```python
from build123d import *

# Parameters (mm, degrees)
SKETCH_1_R               = 28.5
SKETCH_1_R_2             = 21.75
EXTRUDE_1_DEPTH          = 8
CHAMFER_1_SIZE           = 1
CHAMFER_2_SIZE           = 0.5
CUT_EXTRUDE_START        = -8
CUT_EXTRUDE_1_DEPTH      = 8
PATTERN_CIRCULAR_1_COUNT = 4


with BuildPart() as part:
    # 草图1 → 凸台-拉伸1 (new body)
    with BuildSketch(Plane(origin=(0, 0, 0), x_dir=(0, 0, -1), z_dir=(1, 0, 0))):
        Circle(SKETCH_1_R)
        Circle(SKETCH_1_R_2, mode=Mode.SUBTRACT)
    extrude(amount=EXTRUDE_1_DEPTH)

    # 倒角1
    chamfer_1_edges = [part.edges().sort_by_distance(p)[0] for p in [
        (0, 0, 21.75),
        (8, 0, 21.75),
    ]]
    chamfer(chamfer_1_edges, length=CHAMFER_1_SIZE)

    # 倒角2
    chamfer_2_edges = [part.edges().sort_by_distance(p)[0] for p in [
        (0, 0, 28.5),
    ]]
    chamfer(chamfer_2_edges, length=CHAMFER_2_SIZE)

    # 草图2 → 切除-拉伸1 (cut)
    with BuildSketch(Plane(origin=(8, 0, 0), x_dir=(0, 0, -1), z_dir=(1, 0, 0)).offset(CUT_EXTRUDE_START)):
        with BuildLine():
            Line((-3, 28.341665442), (-3, 26.5))
            Line((-3, 26.5), (3, 26.5))
            Line((3, 26.5), (3, 28.341665442))
            ThreePointArc((3, 28.341665442), (0, 28.5), (-3, 28.341665442))
        make_face()
    cut_extrude_1 = extrude(amount=CUT_EXTRUDE_1_DEPTH, mode=Mode.SUBTRACT)

    # 阵列(圆周)1: 切除-拉伸1 ×4 about axis
    pattern_circular_1_axis = Axis((0, 0, 0), (1, 0, 0))
    for i in range(1, PATTERN_CIRCULAR_1_COUNT):
        add(cut_extrude_1.rotate(pattern_circular_1_axis, i * 360 / PATTERN_CIRCULAR_1_COUNT), mode=Mode.SUBTRACT)

    # 草图3 → 切除-旋转1 (revolve, cut)
    with BuildSketch(Plane.XY, mode=Mode.PRIVATE) as cut_revolve_1_sk:
        Polygon((3.295131606, 35.18962283), (8, 25.1), (8, 35.18962283), align=None)
    revolve(cut_revolve_1_sk.sketch.rotate(Axis((8, 0, 0), (-1, 0, 0)), 276.042328419), axis=Axis((8, 0, 0), (-1, 0, 0)), mode=Mode.SUBTRACT)


solid = part.part
```
For this review, take the finished solid that the model builds, in its own axes (mm). A direction names the side the tool comes from. Give positions to 0.01 mm unless a question says otherwise; leave off trailing zeros. Order: outer loops, then holes, each group sorted by start corner. A loop starts at its lowest first (then second) coordinate and runs counter-clockwise, first axis right, second up.
1) Take a section at A-A (z = 0). Give the boundary of the cut face in (x, y).
2) Take a section at C-C (x = 3). Give the boundary of the cut face in (y, z), then the cut area to 3 significant figures.
3) The part is to be moulded in two halves that separate along Z. For faces 5 (the face through (4, 3, -27)), 6 (the face through (4, -26.5, 0)), 7 (the face through (3.416, 19.96, -20.343)), say which applies: released by +Z, released by -Z, zero draft, split by the parting line, or undercut.
4) Wall thickness on line 1 (Y direction, x = 5.4, z = 0); line 2 (Z direction, x = 6, y = 20); line 3 (Z direction, x = 2.5, y = 3.5): over which ranges is each line inside the solid? List them lowest first.
5) For faces 1 (the face through (4, -3, 27)), 2 (the face through (4, -3, -27)), 3 (the face through (4, -27, 3)), 4 (the face through (4, 26.5, 0)), list the 3-axis set-ups (+Z, -Z, +X, -X, +Y, -Y) from which the entire face can be reached by the end or side of a thin tool; tool diameter is ignored.
6) Insertion check: pin 1 (3 mm diameter, centred on x = 3, z = 0.5, fed in from -Y); pin 2 (1.8 mm diameter, centred on x = 2, y = 1.5, fed in from +Z); pin 3 (2 mm diameter, centred on x = 2, y = 27, fed in from -Z). Each pin has a flat end and moves straight along its axis. Give the tip position at first contact, or say it passes through.
Derived:
1. outline: (0, -26.5) - (7.35, -26.5) - (8, -25.1) - (8, -22.75) - (7, -21.75) - (1, -21.75) - (0, -22.75) - close; (0, 22.75) - (1, 21.75) - (7, 21.75) - (8, 22.75) - (8, 25.1) - (7.35, 26.5) - (0, 26.5) - close
2. outline: (-28.34, -3) arc R28.5 ccw to (-3, -28.34) - (-3, -26.5) - (3, -26.5) - (3, -28.34) arc R28.5 ccw to (28.34, -3) - (26.5, -3) - (26.5, 3) - (28.34, 3) arc R28.5 ccw to (3, 28.34) - (3, 26.5) - (-3, 26.5) - (-3, 28.34) arc R28.5 ccw to (-28.34, 3) - (-26.5, 3) - (-26.5, -3) - close; hole circle Ø43.5 at (0, 0)
2. area: 1,020 mm2
3. face 5: zero draft
3. face 6: undercut
3. face 7: released by -Z
4. line 1: y = -26.5 to -21.75, 21.75 to 26.5
4. line 2: z = -20.3 to -8.55, 8.55 to 20.3
4. line 3: z = -28.28 to -21.47, 21.47 to 28.28
5. face 1: +Z, +X, -X
5. face 2: -Z, +X, -X
5. face 3: +X, -X, -Y
5. face 4: +X, -X, +Y
6. pin 1: stops at y = -26.5
6. pin 2: stops at z = 26.5
6. pin 3: stops at z = -11.67
